Source: CAD feature listing. Evaluate the final solid. Frame: model axes, mm. Coordinates: 2 decimals unless noted, no trailing zeros. One line per question, with ' | ' between items. Start each with the question number.
```python
from build123d import *

# Parameters (mm, degrees)
SKETCH5_R          = 75.245114963
SKETCH5_R_2        = 60.176466442
CUT_EXTRUDE1_DEPTH = 10


with BuildPart() as part:
    # Sketch1 → Loft4 section 0
    with BuildSketch(Plane(origin=(0, 0, 0), x_dir=(0, 0, -1), z_dir=(1, 0, 0))):
        Polygon((-205, 200), (195, 200), (195, 190), (0, 190), (0, -190), (195, -190), (195, -200), (-205, -200), (-205, -190), (-10, -190), (-10, 190), (-205, 190), align=None)
    # Sketch4 → Loft4 section 1
    with BuildSketch(Plane(origin=(1000, 0, -1000), x_dir=(0, 0, 1), z_dir=(-1, 0, 0))):
        Polygon((880, 100), (1130, 100), (1130, 90), (1010, 90), (1010, -90), (1130, -90), (1130, -100), (880, -100), (880, -90), (1000, -90), (1000, 90), (880, 90), align=None)
    loft()

    # Sketch5 → Cut-Extrude1 (cut)
    with BuildSketch(Plane.XY.offset(10)):
        with Locations((186.377200583, 0)):
            Circle(SKETCH5_R)
        with Locations((407.046905619, 0)):
            Circle(SKETCH5_R_2)
    extrude(amount=-CUT_EXTRUDE1_DEPTH, mode=Mode.SUBTRACT)


solid = part.part
```
(1) Draft query along Y for faces 1 (the cylindrical face through (111.205, 3.308, 5.07)), 2 (the flat face through (0, 2, 5)). Return one class per face: pulls with the +Y half, pulls with the -Y half, needs draft (parallel to the pull), parting line crosses it, or undercut.
(2) Contact query for flat-ended pins moving along their axis: pin 1 Ø5 at (x, z) = (181, -13.5) entering from -Y; pin 2 Ø5 at (x, z) = (254, 104.5) entering from -Y; pin 3 Ø2 at (x, y) = (277, 97.5) entering from -Z. Output: stop coordinate, or through.
(3) Ray query, L1, parallel to Z at x = 248, y = 72.5; L2, parallel to Y at x = 420.5, z = -29; L3, parallel to Y at x = 797, z = -77. Return the intervals inside material, ascending.
(4) Cut plane A-A, the plane y = 0. State how many separate pieces and enclosed holes the cut face has, and give its area (3 significant figures).
Here are the results:
1) face 1: undercut | face 2: needs draft
2) pin 1: stops at y = -182.15 | pin 2: stops at y = -174.85 | pin 3: stops at z = 0
3) L1: z = 0 to 10 | L2: y = -157.95 to -147.95, 147.95 to 157.95 | L3: y = -120.3 to -110.3, 110.3 to 120.3
4) separate pieces: 3 | enclosed holes: 0 | area: 7,290 mm2
